```python
from build123d import *

# Parameters (mm, degrees)
PCB_STAND_DEPTH     = 30.5
SKETCH3_W           = 95
SKETCH3_H           = 7
EXTRA_BOTTOM_DEPTH  = 2
SENSOR_HOLES_2_R    = 4.6
SENSOR_HOLES_2_R_2  = 4
SENSOR_HOLES_DEPTH  = 58.97844427
SKETCH4_R           = 5.5
SKETCH4_R_2         = 4.5
SENSOR_STANDS_DEPTH = 3.5
FILLET1_R           = 3
SKETCH5_W           = 3
SKETCH5_H           = 0.75
TOF_SLOT_DEPTH      = 1.5


with BuildPart() as part:
    # Master_Geometry → PCB_Stand (new, symmetric)
    with BuildSketch(Plane.XY):
        Polygon((-47.5, -5), (-47.5, 0), (-45.5, 0), (-45.5, -1.5), (-43.5, -1.5), (-43.5, -5), (43.5, -5), (43.5, -1.5), (45.5, -1.5), (45.5, 0), (47.5, 0), (47.5, -5), (47.5, -7), (-47.5, -7), align=None)
    extrude(amount=PCB_STAND_DEPTH, both=True)

    # Sketch3 → Extra_Bottom (add)
    with BuildSketch(Plane.XY.offset(30.5)):
        with Locations((0, -3.5)):
            Rectangle(SKETCH3_W, SKETCH3_H)
    extra_bottom = extrude(amount=EXTRA_BOTTOM_DEPTH)

    # Mirror2: Extra_Bottom across plane
    add(extra_bottom.mirror(Plane.XY))

    # Sensor-Holes 2 → Sensor_Holes (cut, through all)
    with BuildSketch(Plane.XZ.offset(7)):
        with Locations((-37.5, 0)):
            Circle(SENSOR_HOLES_2_R)
        with Locations((20.5, 0)):
            Circle(SENSOR_HOLES_2_R_2)
    extrude(amount=-SENSOR_HOLES_DEPTH, mode=Mode.SUBTRACT)

    # Sketch4 → Sensor_Stands (add)
    # profile 1 of 2: a face of its own
    with BuildSketch(Plane(origin=(0, -5, 0), x_dir=(1, 0, 0), z_dir=(0, 1, 0))):
        with Locations(Location((20.5, 0, 0), (0, 0, 90))):
            Circle(SKETCH4_R)
        with BuildLine():
            Line((16.517616919, 0.375), (24.482383081, 0.375))
            ThreePointArc((24.482383081, 0.375), (20.5, 4), (16.517616919, 0.375))
        make_face(mode=Mode.SUBTRACT)
        with BuildLine():
            Line((16.517616919, -0.375), (24.482383081, -0.375))
            ThreePointArc((24.482383081, -0.375), (20.5, -4), (16.517616919, -0.375))
        make_face(mode=Mode.SUBTRACT)
    # profile 2 of 2: a face of its own
    with BuildSketch(Plane(origin=(0, -5, 0), x_dir=(1, 0, 0), z_dir=(0, 1, 0))):
        with BuildLine():
            Line((-43.5, 14.361406616), (-43.5, -14.361406616))
            ThreePointArc((-43.5, -14.361406616), (-41.534384236, -9.109149302), (-36.603448276, -6.437871931))
            ThreePointArc((-36.603448276, -6.437871931), (-31, 0), (-36.603448276, 6.437871931))
            ThreePointArc((-36.603448276, 6.437871931), (-41.534384236, 9.109149302), (-43.5, 14.361406616))
        make_face()
        with Locations(Location((-37.5, 0, 0), (0, 0, 90))):
            Circle(SKETCH4_R_2, mode=Mode.SUBTRACT)
    extrude(amount=SENSOR_STANDS_DEPTH)

    # Fillet1
    fillet1_edges = [part.edges().sort_by_distance(p)[0] for p in [
        (-41.534384236, -5, 9.109149302),
        (-31, -5, 0),
        (-41.534384236, -5, -9.109149302),
        (0, -5, -30.5),
        (-43.5, -5, 22.430703308),
        (43.5, -5, 0),
        (0, -5, 30.5),
        (20.5, -5, 5.5),
        (-43.5, -5, -22.430703308),
    ]]
    fillet(fillet1_edges, radius=FILLET1_R)

    # Sketch5 → ToF_Slot (cut)
    with BuildSketch(Plane(origin=(0, -1.5, 0), x_dir=(1, 0, 0), z_dir=(0, 1, 0))):
        with Locations((20.5, 0)):
            Rectangle(SKETCH5_W, SKETCH5_H)
    extrude(amount=-TOF_SLOT_DEPTH, mode=Mode.SUBTRACT)


solid = part.part
```
Model file for the job. Use its own axes, mm. A direction names the side the tool comes from. Coordinates: 2 decimals unless noted, no trailing zeros. Order: outer loops, then holes, each group sorted by start corner. A loop starts at its lowest first (then second) coordinate and runs counter-clockwise, first axis right, second up. Notation, with made-up numbers: (77.25, 6.5) -> (102.25, 6.5) arc R34 cw to (102.25, 41.5) -> close; hole circle Ø9 at (-10.5, 43). An arc over 180 degrees is marked (long way). Answer as a JSON object with one key per item and string values. Group by question number.
1) Cut at A-A, the plane y = -4. Write the cut outline in (x, z) (1 decimal).
2) Cut at B-B, the plane x = 20.5. Write the cut outline in (y, z) (3 decimals), then the cut area to 3 significant figures.
3) Which spindle directions (+Z, -Z, +X, -X, +Y, -Y) get a long thin tool onto all of the face, cutting with end or side? Do faces 1 (the face through (-33.11, -6.01, 1.38)), 2 (the face through (-4, 0, -31)), 3 (the face through (44, -1.5, 0)), 4 (the face through (-1, -7, 0)), 5 (the face through (20.4, -3.3, 0.375)). Say none if no direction does.
4) Flat gauge pins, fed straight in: pin 1 (3 mm diameter, centred on x = -18, z = 13, fed in from +Y); pin 2 (0.8 mm diameter, centred on x = 20.5, z = 0, fed in from -Y); pin 3 (10.5 mm diameter, centred on x = -37.5, z = 0, fed in from +Y). Where does each tip first touch, or does it go through?
5) Cut at C-C, the plane x = -5.5. Write the cut outline in (y, z).
6) Cut at D-D, the plane z = 2. Count the separate pieces of the cut face and the enclosed holes in it, then the cut area to 3 significant figures.
7) Pull direction Z, two halves, no side cores. Call faces 6 (the face through (-33.11, -3.27, 0.98)), 7 (the face through (-42.6, -4.14, -22.54)), 8 (the face through (-47.5, -4, 0)): +Z half, -Z half, draft (parallel to the pull), parting line (faces both ways), or undercut.
8) Drill centre lines: L1, parallel to Z at x = 20.5, y = -6.4; L2, parallel to Z at x = -6.5, y = -1.5; L3, parallel to X at y = -1, z = -4. Where is each one in solid material? Low to high.
Check values:
{
 "1": {"outline": "(-47.5, -32.5) -> (47.5, -32.5) -> (47.5, 32.5) -> (-47.5, 32.5) -> close; circle Ø12.5 at (20.5, 0); hole (-42.7, -29.7) -> (42.7, -29.7) -> (42.7, 29.7) -> (-42.7, 29.7) -> (-42.7, 14.4) arc R7.2 ccw to (-36.5, 7.2) arc R7.3 cw to (-36.5, -7.2) arc R7.2 ccw to (-42.7, -14.4) -> close; hole circle Ø9 at (-37.5, 0); hole (16.5, -0.4) arc R4 ccw to (24.5, -0.4) -> close; hole (16.5, 0.4) -> (24.5, 0.4) arc R4 ccw to start"},
 "2": {"outline": "(-7, -32.5) -> (0, -32.5) -> (0, -30.5) -> (-2, -30.5) arc R3 cw to (-5, -27.5) -> (-5, -8.5) arc R3 cw to (-2, -5.5) -> (-1.5, -5.5) -> (-1.5, -4) -> (-7, -4) -> close; (-7, 4) -> (-1.5, 4) -> (-1.5, 5.5) -> (-2, 5.5) arc R3 cw to (-5, 8.5) -> (-5, 27.5) arc R3 cw to (-2, 30.5) -> (0, 30.5) -> (0, 32.5) -> (-7, 32.5) -> close; (-5, -0.375) -> (-3, -0.375) -> (-3, 0.375) -> (-5, 0.375) -> close", "area": "154 mm²"},
 "3": {"face 1": "-Y", "face 2": "+Z, -Z, +X, -X, +Y", "face 3": "+Y", "face 4": "+Z, -Z, +X, -X, -Y", "face 5": "+Y, -Y"},
 "4": {"pin 1": "stops at y = -5", "pin 2": "stops at y = -5", "pin 3": "stops at y = -1.5"},
 "5": {"outline": "(-7, -32.5) -> (0, -32.5) -> (0, -30.5) -> (-2, -30.5) arc R3 cw to (-5, -27.5) -> (-5, 27.5) arc R3 cw to (-2, 30.5) -> (0, 30.5) -> (0, 32.5) -> (-7, 32.5) -> close"},
 "6": {"separate pieces": "3", "enclosed holes": "0", "area": "228 mm²"},
 "7": {"face 6": "undercut", "face 7": "undercut", "face 8": "draft"},
 "8": {"L1": "z = -32.5 to -4, 4 to 32.5", "L2": "z = -32.5 to -30.5, 30.5 to 32.5", "L3": "x = -47.5 to -45.5, 45.5 to 47.5"}
}
